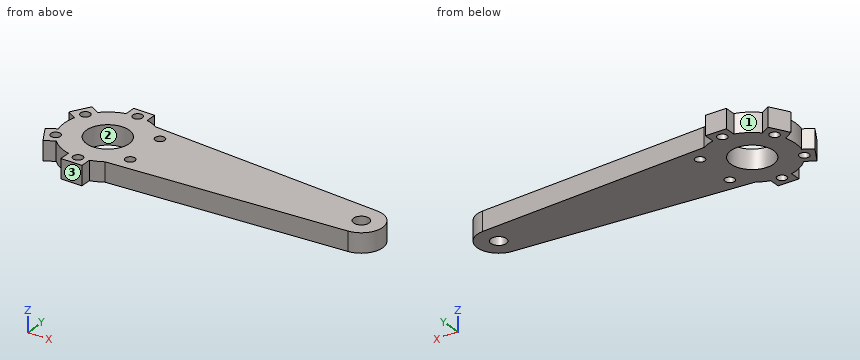
from build123d import *

# Parameters (mm, degrees)
SKETCH_1_R      = 2.5
SKETCH_1_R_2    = 11.05
SKETCH_1_R_3    = 4
EXTRUDE_1_DEPTH = 10


with BuildPart() as part:
    # 草图1 → 凸台-拉伸1 (new body)
    with BuildSketch(Plane.XY):
        with BuildLine():
            ThreePointArc((11.821054836, 19.144520432), (8.76303822, 20.723396468), (5.5, 21.817424229))
            Line((5.5, 21.817424229), (5.5, 27.5))
            Line((5.5, 27.5), (-5.5, 27.5))
            Line((-5.5, 27.5), (-5.5, 21.817424229))
            ThreePointArc((-5.5, 21.817424229), (-11.25, 19.485571585), (-16.144443628, 15.671851835))
            Line((-16.144443628, 15.671851835), (-21.065698604, 18.513139721))
            Line((-21.065698604, 18.513139721), (-26.565698604, 8.986860279))
            Line((-26.565698604, 8.986860279), (-21.644443628, 6.145572394))
            ThreePointArc((-21.644443628, 6.145572394), (-22.5, 0), (-21.644443628, -6.145572394))
            Line((-21.644443628, -6.145572394), (-26.565698604, -8.986860279))
            Line((-26.565698604, -8.986860279), (-21.065698604, -18.513139721))
            Line((-21.065698604, -18.513139721), (-16.144443628, -15.671851835))
            ThreePointArc((-16.144443628, -15.671851835), (-11.25, -19.485571585), (-5.5, -21.817424229))
            Line((-5.5, -21.817424229), (-5.5, -27.5))
            Line((-5.5, -27.5), (5.5, -27.5))
            Line((5.5, -27.5), (5.5, -21.817424229))
            ThreePointArc((5.5, -21.817424229), (8.76303822, -20.723396468), (11.821054836, -19.144520432))
            Line((11.821054836, -19.144520432), (133.336666591, -11.0254171))
            ThreePointArc((133.336666591, -11.0254171), (143.649999924, 0), (133.336666591, 11.0254171))
            Line((133.336666591, 11.0254171), (11.821054836, 19.144520432))
        make_face()
        with Locations((19.485571585, -11.25)):
            Circle(SKETCH_1_R, mode=Mode.SUBTRACT)
        with Locations((19.485571585, 11.25)):
            Circle(SKETCH_1_R, mode=Mode.SUBTRACT)
        with Locations((-19.485571585, -11.25)):
            Circle(SKETCH_1_R, mode=Mode.SUBTRACT)
        with Locations((-19.485571585, 11.25)):
            Circle(SKETCH_1_R, mode=Mode.SUBTRACT)
        with Locations((0, -22.5)):
            Circle(SKETCH_1_R, mode=Mode.SUBTRACT)
        with Locations((0, 22.5)):
            Circle(SKETCH_1_R, mode=Mode.SUBTRACT)
        Circle(SKETCH_1_R_2, mode=Mode.SUBTRACT)
        with Locations((132.599999924, 0)):
            Circle(SKETCH_1_R_3, mode=Mode.SUBTRACT)
    extrude(amount=EXTRUDE_1_DEPTH)


solid = part.part
Can you work these out from the model? Positions are in its coordinate system, mm. Face numbers are marked on the shaded views. Give positions to 0.01 mm unless a question says otherwise; leave off trailing zeros. Order: outer loops, then holes, each group sorted by start corner. A loop starts at its lowest first (then second) coordinate and runs counter-clockwise, first axis right, second up. Notation, with made-up numbers: (30.25, 74.25) - (67.25, 74.25) arc R14 ccw to (67.25, 99.25) - close; hole circle Ø7 at (88, -28.5). An arc over 180 degrees is marked (long way). Write each question's results on one line, items separated by ' | '.
1) If we mould it in two halves opening along Y, with no side actions, what happens to the marked faces 1, 2 and 3? For each: pulls with the +Y half, pulls with the -Y half, needs draft (parallel to the pull), parting line crosses it, or undercut.
Final values:
face 1: pulls with the +Y half | face 2: undercut | face 3: pulls with the -Y half
2) Suppose I cut it at A-A, the plane x = 0. Write out the boundary of the cut face in (y, z), then the cut area to 3 significant figures.
Final values:
outline: (-27.5, 0) - (-25, 0) - (-25, 10) - (-27.5, 10) - close; (-20, 0) - (-11.05, 0) - (-11.05, 10) - (-20, 10) - close; (11.05, 0) - (20, 0) - (20, 10) - (11.05, 10) - close; (25, 0) - (27.5, 0) - (27.5, 10) - (25, 10) - close | area: 229 mm^2
3) Suppose I cut it at B-B, the plane z = 6.5. Give the number of separate pieces and of enclosed holes in the cut face, then the cut area to 3 significant figures.
Final values:
separate pieces: 1 | enclosed holes: 8 | area: 4,820 mm^2
4) I'm going to push flat-ended pins straight in: pin 1 Ø3 at (y, z) = (-24.5, 4) entering from +X; pin 2 Ø4.5 at (y, z) = (-24.5, 6) entering from -X; pin 3 Ø3 at (x, z) = (86, 7.5) entering from -Y; pin 4 Ø8 at (x, y) = (-19.49, -11.25) entering from +Z. Where does each tip first touch, or does it pass through?
Final values:
pin 1: stops at x = 5.5 | pin 2: stops at x = -5.5 | pin 3: stops at y = -14.29 | pin 4: stops at z = 10
5) Please list where these lines run through material, in increasing order: line 1 along Y through (x, z) = (132.6, 3.25); line 2 along Y through (x, z) = (0, 7.5); line 3 along X through (y, z) = (1.5, 1.25). Write a range as [from, to].
Final values:
line 1: y = [-11.07, -4], [4, 11.07] | line 2: y = [-27.5, -25], [-20, -11.05], [11.05, 20], [25, 27.5] | line 3: x = [-22.45, -10.95], [10.95, 128.89], [136.31, 143.55]
6) Suppose I cut it at C-C, the plane x = 24.5. Write out the boundary of the cut face in (y, z).
Final values:
outline: (-18.3, 0) - (18.3, 0) - (18.3, 10) - (-18.3, 10) - close
